Can you work these out from the model? Positions are in its coordinate system, mm. Round coordinates to 2 decimals unless told otherwise and drop trailing zeros. Answer as a JSON object with one key per item and string values. Group by question number.
```python
from build123d import *

# Parameters (mm, degrees)
SKETCH_1_W          = 90
SKETCH_1_H          = 90
EXTRUDE_1_DEPTH     = 3
SKETCH_2_R          = 1.5
CUT_EXTRUDE_1_DEPTH = 64.710281745
SKETCH_3_R          = 1.5
CUT_EXTRUDE_2_DEPTH = 64.710281745
SKETCH_5_R          = 1.5
CUT_EXTRUDE_3_DEPTH = 64.710281745
FILLET_1_R          = 4
SKETCH_6_R          = 2.1
CUT_EXTRUDE_5_DEPTH = 64.710281745


with BuildPart() as part:
    # 草图1 → 凸台-拉伸1 (new body)
    with BuildSketch(Plane(origin=(0, 0, 0), x_dir=(1, 0, 0), z_dir=(0, 1, 0))):
        Rectangle(SKETCH_1_W, SKETCH_1_H)
    extrude(amount=EXTRUDE_1_DEPTH)

    # 草图2 → 切除-拉伸1 (cut, through all)
    with BuildSketch(Plane(origin=(0, 3, 0), x_dir=(1, 0, 0), z_dir=(0, 1, 0))):
        with Locations(Location((-40, 40, 0), (0, 0, 270))):
            Circle(SKETCH_2_R)
        with Locations(Location((40, 40, 0), (0, 0, 270))):
            Circle(SKETCH_2_R)
        with Locations(Location((40, -40, 0), (0, 0, 270))):
            Circle(SKETCH_2_R)
        with Locations(Location((-40, -40, 0), (0, 0, 270))):
            Circle(SKETCH_2_R)
    extrude(amount=-CUT_EXTRUDE_1_DEPTH, mode=Mode.SUBTRACT)

    # 草图3 → 切除-拉伸2 (cut, through all)
    with BuildSketch(Plane(origin=(0, 3, 0), x_dir=(1, 0, 0), z_dir=(0, 1, 0))):
        with Locations(Location((0, 0, 0), (0, 0, 270))):
            Circle(SKETCH_3_R)
        with Locations(Location((10, 0, 0), (0, 0, 270))):
            Circle(SKETCH_3_R)
        with Locations(Location((20, 0, 0), (0, 0, 270))):
            Circle(SKETCH_3_R)
        with Locations(Location((30, 0, 0), (0, 0, 270))):
            Circle(SKETCH_3_R)
        with Locations(Location((40, 0, 0), (0, 0, 270))):
            Circle(SKETCH_3_R)
        with Locations(Location((10, 10, 0), (0, 0, 270))):
            Circle(SKETCH_3_R)
        with Locations(Location((30, 10, 0), (0, 0, 270))):
            Circle(SKETCH_3_R)
        with Locations(Location((40, 10, 0), (0, 0, 270))):
            Circle(SKETCH_3_R)
        with Locations(Location((10, 20, 0), (0, 0, 270))):
            Circle(SKETCH_3_R)
        with Locations(Location((20, 20, 0), (0, 0, 270))):
            Circle(SKETCH_3_R)
        with Locations(Location((30, 20, 0), (0, 0, 270))):
            Circle(SKETCH_3_R)
        with Locations(Location((40, 20, 0), (0, 0, 270))):
            Circle(SKETCH_3_R)
        with Locations(Location((10, 30, 0), (0, 0, 270))):
            Circle(SKETCH_3_R)
        with Locations(Location((20, 30, 0), (0, 0, 270))):
            Circle(SKETCH_3_R)
        with Locations(Location((30, 30, 0), (0, 0, 270))):
            Circle(SKETCH_3_R)
        with Locations(Location((40, 30, 0), (0, 0, 270))):
            Circle(SKETCH_3_R)
        with Locations(Location((10, 40, 0), (0, 0, 270))):
            Circle(SKETCH_3_R)
        with Locations(Location((20, 40, 0), (0, 0, 270))):
            Circle(SKETCH_3_R)
        with Locations(Location((30, 40, 0), (0, 0, 270))):
            Circle(SKETCH_3_R)
        with Locations(Location((40, 40, 0), (0, 0, 270))):
            Circle(SKETCH_3_R)
        with Locations(Location((0, 10, 0), (0, 0, 270))):
            Circle(SKETCH_3_R)
        with Locations(Location((0, 30, 0), (0, 0, 270))):
            Circle(SKETCH_3_R)
        with Locations(Location((0, 40, 0), (0, 0, 270))):
            Circle(SKETCH_3_R)
        with Locations(Location((-10, 0, 0), (0, 0, 270))):
            Circle(SKETCH_3_R)
        with Locations(Location((-20, 0, 0), (0, 0, 270))):
            Circle(SKETCH_3_R)
        with Locations(Location((-30, 0, 0), (0, 0, 270))):
            Circle(SKETCH_3_R)
        with Locations(Location((-40, 0, 0), (0, 0, 270))):
            Circle(SKETCH_3_R)
        with Locations(Location((-10, -10, 0), (0, 0, 270))):
            Circle(SKETCH_3_R)
        with Locations(Location((-30, -10, 0), (0, 0, 270))):
            Circle(SKETCH_3_R)
        with Locations(Location((-40, -10, 0), (0, 0, 270))):
            Circle(SKETCH_3_R)
        with Locations(Location((-10, -20, 0), (0, 0, 270))):
            Circle(SKETCH_3_R)
        with Locations(Location((-20, -20, 0), (0, 0, 270))):
            Circle(SKETCH_3_R)
        with Locations(Location((-30, -20, 0), (0, 0, 270))):
            Circle(SKETCH_3_R)
        with Locations(Location((-40, -20, 0), (0, 0, 270))):
            Circle(SKETCH_3_R)
        with Locations(Location((-10, -30, 0), (0, 0, 270))):
            Circle(SKETCH_3_R)
        with Locations(Location((-20, -30, 0), (0, 0, 270))):
            Circle(SKETCH_3_R)
        with Locations(Location((-30, -30, 0), (0, 0, 270))):
            Circle(SKETCH_3_R)
        with Locations(Location((-40, -30, 0), (0, 0, 270))):
            Circle(SKETCH_3_R)
        with Locations(Location((-10, -40, 0), (0, 0, 270))):
            Circle(SKETCH_3_R)
        with Locations(Location((-20, -40, 0), (0, 0, 270))):
            Circle(SKETCH_3_R)
        with Locations(Location((-30, -40, 0), (0, 0, 270))):
            Circle(SKETCH_3_R)
        with Locations(Location((-40, -40, 0), (0, 0, 270))):
            Circle(SKETCH_3_R)
        with Locations(Location((0, -10, 0), (0, 0, 270))):
            Circle(SKETCH_3_R)
        with Locations(Location((0, -30, 0), (0, 0, 270))):
            Circle(SKETCH_3_R)
        with Locations(Location((0, -40, 0), (0, 0, 270))):
            Circle(SKETCH_3_R)
    extrude(amount=-CUT_EXTRUDE_2_DEPTH, mode=Mode.SUBTRACT)

    # 草图5 → 切除-拉伸3 (cut, through all)
    with BuildSketch(Plane(origin=(0, 3, 0), x_dir=(1, 0, 0), z_dir=(0, 1, 0))):
        with Locations(Location((0, 0, 0), (0, 0, 270))):
            Circle(SKETCH_5_R)
        with Locations(Location((-10, 0, 0), (0, 0, 270))):
            Circle(SKETCH_5_R)
        with Locations(Location((-20, 0, 0), (0, 0, 270))):
            Circle(SKETCH_5_R)
        with Locations(Location((-30, 0, 0), (0, 0, 270))):
            Circle(SKETCH_5_R)
        with Locations(Location((-40, 0, 0), (0, 0, 270))):
            Circle(SKETCH_5_R)
        with Locations(Location((-10, 10, 0), (0, 0, 270))):
            Circle(SKETCH_5_R)
        with Locations(Location((-30, 10, 0), (0, 0, 270))):
            Circle(SKETCH_5_R)
        with Locations(Location((-40, 10, 0), (0, 0, 270))):
            Circle(SKETCH_5_R)
        with Locations(Location((-10, 20, 0), (0, 0, 270))):
            Circle(SKETCH_5_R)
        with Locations(Location((-20, 20, 0), (0, 0, 270))):
            Circle(SKETCH_5_R)
        with Locations(Location((-30, 20, 0), (0, 0, 270))):
            Circle(SKETCH_5_R)
        with Locations(Location((-40, 20, 0), (0, 0, 270))):
            Circle(SKETCH_5_R)
        with Locations(Location((-10, 30, 0), (0, 0, 270))):
            Circle(SKETCH_5_R)
        with Locations(Location((-20, 30, 0), (0, 0, 270))):
            Circle(SKETCH_5_R)
        with Locations(Location((-30, 30, 0), (0, 0, 270))):
            Circle(SKETCH_5_R)
        with Locations(Location((-40, 30, 0), (0, 0, 270))):
            Circle(SKETCH_5_R)
        with Locations(Location((-10, 40, 0), (0, 0, 270))):
            Circle(SKETCH_5_R)
        with Locations(Location((-20, 40, 0), (0, 0, 270))):
            Circle(SKETCH_5_R)
        with Locations(Location((-30, 40, 0), (0, 0, 270))):
            Circle(SKETCH_5_R)
        with Locations(Location((-40, 40, 0), (0, 0, 270))):
            Circle(SKETCH_5_R)
        with Locations(Location((0, 10, 0), (0, 0, 270))):
            Circle(SKETCH_5_R)
        with Locations(Location((0, 30, 0), (0, 0, 270))):
            Circle(SKETCH_5_R)
        with Locations(Location((0, 40, 0), (0, 0, 270))):
            Circle(SKETCH_5_R)
        with Locations(Location((10, 0, 0), (0, 0, 270))):
            Circle(SKETCH_5_R)
        with Locations(Location((20, 0, 0), (0, 0, 270))):
            Circle(SKETCH_5_R)
        with Locations(Location((30, 0, 0), (0, 0, 270))):
            Circle(SKETCH_5_R)
        with Locations(Location((40, 0, 0), (0, 0, 270))):
            Circle(SKETCH_5_R)
        with Locations(Location((10, -10, 0), (0, 0, 270))):
            Circle(SKETCH_5_R)
        with Locations(Location((30, -10, 0), (0, 0, 270))):
            Circle(SKETCH_5_R)
        with Locations(Location((40, -10, 0), (0, 0, 270))):
            Circle(SKETCH_5_R)
        with Locations(Location((10, -20, 0), (0, 0, 270))):
            Circle(SKETCH_5_R)
        with Locations(Location((20, -20, 0), (0, 0, 270))):
            Circle(SKETCH_5_R)
        with Locations(Location((30, -20, 0), (0, 0, 270))):
            Circle(SKETCH_5_R)
        with Locations(Location((40, -20, 0), (0, 0, 270))):
            Circle(SKETCH_5_R)
        with Locations(Location((10, -30, 0), (0, 0, 270))):
            Circle(SKETCH_5_R)
        with Locations(Location((20, -30, 0), (0, 0, 270))):
            Circle(SKETCH_5_R)
        with Locations(Location((30, -30, 0), (0, 0, 270))):
            Circle(SKETCH_5_R)
        with Locations(Location((40, -30, 0), (0, 0, 270))):
            Circle(SKETCH_5_R)
        with Locations(Location((10, -40, 0), (0, 0, 270))):
            Circle(SKETCH_5_R)
        with Locations(Location((20, -40, 0), (0, 0, 270))):
            Circle(SKETCH_5_R)
        with Locations(Location((30, -40, 0), (0, 0, 270))):
            Circle(SKETCH_5_R)
        with Locations(Location((40, -40, 0), (0, 0, 270))):
            Circle(SKETCH_5_R)
        with Locations(Location((0, -10, 0), (0, 0, 270))):
            Circle(SKETCH_5_R)
        with Locations(Location((0, -30, 0), (0, 0, 270))):
            Circle(SKETCH_5_R)
        with Locations(Location((0, -40, 0), (0, 0, 270))):
            Circle(SKETCH_5_R)
    extrude(amount=-CUT_EXTRUDE_3_DEPTH, mode=Mode.SUBTRACT)

    # 圆角1
    fillet_1_edges = [part.edges().sort_by_distance(p)[0] for p in [
        (45, 1.5, 45),
        (-45, 1.5, 45),
        (-45, 1.5, -45),
        (45, 1.5, -45),
    ]]
    fillet(fillet_1_edges, radius=FILLET_1_R)

    # 草图6 → 切除-拉伸5 (cut, through all)
    with BuildSketch(Plane(origin=(0, 3, 0), x_dir=(1, 0, 0), z_dir=(0, 1, 0))):
        with Locations(Location((0, 19, 0), (0, 0, 270))):
            Circle(SKETCH_6_R)
        with Locations(Location((16.454482672, 9.5, 0), (0, 0, 270))):
            Circle(SKETCH_6_R)
        with Locations(Location((16.454482672, -9.5, 0), (0, 0, 270))):
            Circle(SKETCH_6_R)
        with Locations(Location((0, -19, 0), (0, 0, 270))):
            Circle(SKETCH_6_R)
        with Locations(Location((-16.454482672, -9.5, 0), (0, 0, 270))):
            Circle(SKETCH_6_R)
        with Locations(Location((-16.454482672, 9.5, 0), (0, 0, 270))):
            Circle(SKETCH_6_R)
    extrude(amount=-CUT_EXTRUDE_5_DEPTH, mode=Mode.SUBTRACT)


solid = part.part
```
1) I need wall thicknesses on line 1 along Z through (x, y) = (-17, 2.1). Which ranges of the line are inside material? Lowest first, please.
2) We'd pull the mould along Z, two halves only. Please class faces 1 (the face through (-45, 1, 1)), 2 (the face through (9.1, 1.5, -41.2)): +Z half, -Z half, draft (parallel to the pull), parting line (faces both ways), or undercut.
3) If we section it at A-A on z = 0: Count the separate pieces of the cut face and the enclosed holes in it, plus the area to 3 significant figures.
Findings:
{
 "1": {"line 1": "z = -45 to -11.53, -7.47 to 7.47, 11.53 to 45"},
 "2": {"face 1": "draft", "face 2": "undercut"},
 "3": {"separate pieces": "10", "enclosed holes": "0", "area": "189 mm^2"}
}
